Autodesk Inventor part; units mm, degrees
ref_plane "YZ Plane" through (0, 0, 0) normal (1, 0, 0) x (0, 1, 0)
ref_plane "XZ Plane" through (0, 0, 0) normal (0, 1, 0) x (-1, 0, 0)
ref_plane "XY Plane" through (0, 0, 0) normal (0, 0, 1) x (1, 0, 0)
sketch "Sketch1" plane through (0, 0, 0) normal (0, 0, 1) x (1, 0, 0)
  circle A0 centre (4, 0) radius 4
  circle A1 centre (4, 0) radius 3.175
  circle A2 centre (4, 0) radius 3.9492
  circle A3 centre (4, 0) radius 3.2512
  point P0 (0, 0)
  dimension "d0" = 0.0508
  dimension "d1" = 0.0762
extrude "Extrusion1" add sketch "Sketch1" along normal blind 15 and the other way blind 57.0076 contours A2
ref_plane "Work Plane1" through (-7, 0, -17.0076) normal (0, 0, -1) x (-1, 0, 0)
sketch "Sketch2" plane through (-7, 0, -17.0076) normal (0, 0, -1) x (-1, 0, 0)
  circle A0 centre (-11, 0) radius 3.9492
  line L0 (-11, 0) -> (126.5, 0)
  line L1 (-11, 0) -> (-561, 0)
  circle A1 centre (-561, 0) radius 12.7
  circle A2 centre (-11, 0) radius 31.75
  line L2 (35.9, 0) -> (-573.7, 0)
  circle A3 centre (-36.4, 0) radius 2.1
  circle A4 centre (-23.7, -21.997) radius 2.1
  circle A5 centre (1.7, -21.997) radius 2.1
  circle A6 centre (14.4, 0) radius 2.1
  circle A7 centre (1.7, 21.997) radius 2.1
  circle A8 centre (-23.7, 21.997) radius 2.1
  line L3 (1.7, -12.7) -> (-23.7, -12.7)
  line L4 (-23.7, -12.7) -> (-23.7, 12.7)
  line L5 (-23.7, 12.7) -> (1.7, 12.7)
  line L6 (1.7, 12.7) -> (1.7, -12.7)
  line L7 (1.7, -12.7) -> (-23.7, 12.7) construction
  line L8 (-23.7, -12.7) -> (1.7, 12.7) construction
  circle A9 centre (-11, 0) radius 9.525
  point P0 (-7, 0)
  dimension "d8" = 25.4
  dimension "d6" = 137.5
  dimension "d7" = 550
  dimension "d9" = 63.5
  dimension "d10" = 609.6
  dimension "d11" = 4.2
  dimension "d12" = 25.4
  dimension "d15" = 360
  dimension "d17" = 25.4
  dimension "d18" = 25.4
  dimension "d19" = 19.05
extrude "Extrusion2" add sketch "Sketch2" along normal blind 40 contours L0 L1 A0 | L0 A9 L1 A0 | A0 L1 L0 | A0 L1 A9 L0
extrude "Extrusion3" add sketch "Sketch2" along normal blind 10.16 contours L0 L1 A0 | L0 A9 L1 A0 | A0 L1 L0 | A0 L1 A9 L0 | A9 L1 L4 L5 L6 L0 | L0 L6 L3 L4 L1 A9
extrude "Extrusion4" add sketch "Sketch2" along normal blind 3.175 contours L6 L5 L4 L1 A3 A2 L0 A6 | L0 A6 A2 L1 A3 L4 L3 L6
sketch "Sketch3" plane through (4, 0, 15) normal (0, 0, 1) x (1, 0, 0)
  line L0 (8.0047, -6.9197) -> (-11.6012, -6.9197)
  line L1 (-11.6012, -6.9197) -> (-11.6012, 5.9412)
  line L2 (-11.6012, 5.9412) -> (8.0047, 5.9412)
  line L3 (8.0047, 5.9412) -> (8.0047, -6.9197)
  point P0 (-4, 0)
extrude "Extrusion5" cut sketch "Sketch3" against normal blind 32.0076
sketch "Sketch4" plane through (4, 0, -17.0076) normal (0, 0, 1) x (1, 0, 0)
  circle A0 centre (0, 0) radius 3.175
  circle A1 centre (0, 0) radius 3.429
  point P0 (-4, 0)
  dimension "d31" = 0.254
extrude "Extrusion6" cut sketch "Sketch4" against normal blind 40 contours A0 | A1
chamfer "Chamfer2" distance 0.635 angle 45 2 edges at (0.571, 0, -17.0076) (0.571, 0, -57.0076)
properties part number "ArmPivot"
Geometry: final body of the model. Coordinates: model frame, mm. A direction names the side the tool comes from. Coordinates: 2 decimals unless noted, no trailing zeros. Order: outer loops, then holes, each group sorted by start corner. A loop starts at its lowest first (then second) coordinate and runs counter-clockwise, first axis right, second up. Notation, with made-up numbers: M -21.75,64 L 6.25,64 A5 ccw 6.25,70 Z; hole C 57,13 d5. An arc over 180 degrees is marked long. One line per question, with ' | ' between items. Start each with the question number.
Item 1: Set-up query: faces 1 (the flat face through (4, -12.7, -24)), 2 (the cylindrical face through (13.516, -0.419, -41.879)), 3 (the flat face through (-8.7, 0, -24)). Return all of +Z, -Z, +X, -X, +Y, -Y with unobstructed straight access to the full face (end or side cutting, diameter ignored); none if empty.
Item 2: Ray query, probe 1 along Y at (x, z) = (-8.7, -18.6); probe 2 along Y at (x, z) = (16, -18); probe 3 along Z at (x, y) = (16.5, -24.5). Return the intervals inside material, ascending. Write a range as [from, to].
Item 3: Cut plane C-C, the plane x = -10. Return the cut outline in (y, z), then the cut area to 3 significant figures.
Item 4: Pin query (flat end, axial travel): pin 1 Ø6 at (x, y) = (4, 0) entering from -Z; pin 2 Ø5.5 at (x, z) = (1.5, -24.5) entering from +Y; pin 3 Ø8 at (x, y) = (29, -5.5) entering from -Z; pin 4 Ø2 at (x, z) = (1.5, -39) entering from -Y. Return the tip coordinate at first contact, or that it passes through.
Item 5: Cut plane A-A, the plane x = -21.4. Return the cut outline in (y, z), then the cut area to 3 significant figures.
Item 6: Cut plane B-B, the plane y = 0. Return the cut outline in (x, z) (3 decimals).
Item 7: Cut plane D-D, the plane z = -25. Return the cut outline in (x, y), then the cut area to 3 significant figures.
A:
1) face 1: -Z, +X, -X, -Y | face 2: -Z | face 3: -Z, -X, +Y, -Y
2) probe 1: y = [-29.1, -24.1], [-19.9, 19.9], [24.1, 29.1] | probe 2: y = [-29.39, -23.98], [-20.02, 20.02], [23.98, 29.39] | probe 3: z = [-20.18, -17.01]
3) outline: M -28.5,-20.18 L -23.65,-20.18 L -23.65,-17.01 L -28.5,-17.01 Z; M -20.35,-20.18 L 20.35,-20.18 L 20.35,-17.01 L -20.35,-17.01 Z; M 23.65,-20.18 L 28.5,-20.18 L 28.5,-17.01 L 23.65,-17.01 Z | area: 160 mm2
4) pin 1: passes through | pin 2: stops at y = 12.7 | pin 3: stops at z = -20.18 | pin 4: stops at y = -9.41
5) outline: M -19.05,-20.18 L -2.1,-20.18 L -2.1,-17.01 L -19.05,-17.01 Z; M 2.1,-20.18 L 19.05,-20.18 L 19.05,-17.01 L 2.1,-17.01 Z | area: 108 mm2
6) outline: M -27.75,-20.183 L -23.5,-20.183 L -23.5,-17.008 L -27.75,-17.008 Z; M -19.3,-20.183 L -8.7,-20.183 L -8.7,-27.168 L -5.525,-27.168 L -5.525,-57.008 L -0.064,-57.008 L 0.571,-56.373 L 0.571,-17.643 L -0.064,-17.008 L -19.3,-17.008 Z; M 7.429,-56.373 L 8.064,-57.008 L 13.525,-57.008 L 13.525,-27.168 L 16.7,-27.168 L 16.7,-20.183 L 27.3,-20.183 L 27.3,-17.008 L 8.064,-17.008 L 7.429,-17.643 Z; M 31.5,-20.183 L 35.75,-20.183 L 35.75,-17.008 L 31.5,-17.008 Z
7) outline: M -8.7,-12.7 L 16.7,-12.7 L 16.7,12.7 L -8.7,12.7 Z; hole C 4,0 d6.86 | area: 608 mm2
